Verification items for the finished model (mm, model axes). Face numbers are marked on the shaded views. A direction names the side the tool comes from. Give positions to 0.01 mm unless a question says otherwise; leave off trailing zeros. Write each loop counter-clockwise with the first axis right and the second up, starting at its lowest first coordinate (ties: lowest second). Pieces come first, ordered by that corner, then holes. Notation, with made-up numbers: M -31,18 L 25,18 A22 ccw 25,55 Z; hole C 83.5,72.25 d4. An arc over 180 degrees is marked long. Write item = value, one per line.
from build123d import *

# Parameters (mm, degrees)
STOCK_DEPTH        = 9.525
MOUNTING_HOLE_D    = 6.35
SPRING_HOLE_D      = 4.7625
FILLET3_R          = 9.525
FILLET4_R          = 1.27
SKETCH15_W         = 12.7
SKETCH15_H         = 12.7
CUT_EXTRUDE1_DEPTH = 3.175
SKETCH16_W         = 12.7
SKETCH16_H         = 12.7
CUT_EXTRUDE2_DEPTH = 3.175
FILLET5_R          = 3.175


# Some blends are built 0.0001 mm under size
with BuildPart() as part:
    # Sketch7 → Stock (new body)
    with BuildSketch(Plane(origin=(0, 0, 0), x_dir=(1, 0, 0), z_dir=(0, 1, 0))):
        Polygon((0, 0), (0, 19.05), (-7.874, 19.05), (-7.874, 28.575), (6.096, 28.575), (6.096, 69.85), (18.796, 69.85), (18.796, 28.575), (23.876, 28.575), (23.876, 0), align=None)
    extrude(amount=STOCK_DEPTH)

    # Mounting Hole (through all)
    with Locations(Plane(origin=(0, 9.525, 0), x_dir=(1, 0, 0), z_dir=(0, 1, 0))):
        with Locations((14.224, 9.525)):
            Hole(MOUNTING_HOLE_D / 2)

    # Spring Hole (through all)
    with Locations(Plane(origin=(0, 9.525, 0), x_dir=(1, 0, 0), z_dir=(0, 1, 0))):
        with Locations((12.446, 63.5)):
            Hole(SPRING_HOLE_D / 2)

    # Fillet3
    # the kernel refuses this fillet: 9.525 mm, written as the material it adds along each edge
    with BuildSketch(Plane(origin=(6.096, 0, -28.575), x_dir=(-1, 0, 0), z_dir=(0, 1, 0))) as fillet3_piece_1:
        with BuildLine():
            CenterArc((FILLET3_R, -FILLET3_R), FILLET3_R, 90, 90)
            Line((0, -FILLET3_R), (-FILLET3_R * 0.02, -FILLET3_R))
            Line((-FILLET3_R * 0.02, -FILLET3_R), (-FILLET3_R * 0.02, FILLET3_R * 0.02))
            Line((-FILLET3_R * 0.02, FILLET3_R * 0.02), (FILLET3_R, FILLET3_R * 0.02))
            Line((FILLET3_R, FILLET3_R * 0.02), (FILLET3_R, 0))
        make_face()
    extrude(amount=9.525)
    with BuildSketch(Plane(origin=(18.796, 0, -28.575), x_dir=(1, 0, 0), z_dir=(0, 1, 0))) as fillet3_piece_2:
        with BuildLine():
            CenterArc((9.525, 8.424226968), FILLET3_R, 180, 62.181860715)
            Line((0, 8.424226968), (-0.1905, 8.424226968))
            Line((-0.1905, 8.424226968), (-0.1905, 0))
            Line((-0.1905, 0), (0, -0.1905))
            ThreePointArc((0, -0.1905), (2.54, -0.1905), (4.9911, -0.168484539))
            Line((4.9911, -0.168484539), (5.08, 0))
        make_face()
    extrude(amount=9.525)

    # Fillet4
    fillet4_edges = [part.edges().sort_by_distance(p)[0] for p in [
        (-7.874, 4.7625, -28.575),
        (6.096, 4.7625, -69.85),
        (18.796, 4.7625, -69.85),
    ]]
    fillet(fillet4_edges, radius=FILLET4_R)

    # Sketch15 → Cut-Extrude1 (cut)
    with BuildSketch(Plane(origin=(0, 9.525, 0), x_dir=(1, 0, 0), z_dir=(0, 1, 0))):
        with Locations((12.446, 63.5)):
            Rectangle(SKETCH15_W, SKETCH15_H)
    extrude(amount=-CUT_EXTRUDE1_DEPTH, mode=Mode.SUBTRACT)

    # Sketch16 → Cut-Extrude2 (cut)
    with BuildSketch(Plane.XZ):
        with Locations((12.446, -63.5)):
            Rectangle(SKETCH16_W, SKETCH16_H)
    extrude(amount=-CUT_EXTRUDE2_DEPTH, mode=Mode.SUBTRACT)

    # Fillet5
    fillet5_edges = [part.edges().sort_by_distance(p)[0] for p in [
        (12.446, 3.175, -57.15),
        (12.446, 6.35, -57.15),
    ]]
    fillet(fillet5_edges, radius=FILLET5_R - 0.0001)  # a hair under: the kernel refuses the full size


solid = part.part
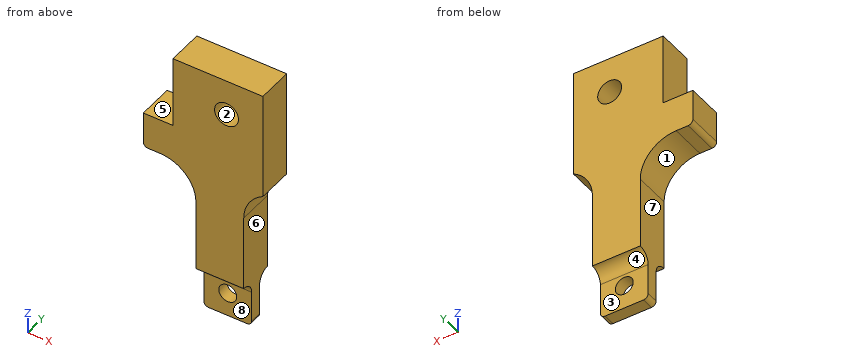
1) Material ranges on probe 1 along X at (y, z) = (5.4, -63.5); probe 2 along Z at (x, y) = (12.5, 5.5); probe 3 along X at (y, z) = (6, -48), recorded low to high. Write a range as from..to.
From the geometry:
probe_1 = 6.1..10.06, 14.83..18.8
probe_2 = -69.85..-65.88, -61.12..-12.19, -6.86..0
probe_3 = 6.1..18.8
2) Tool access check on the marked faces 4, 5, 6, 7 and 8. Record the directions out of +Z, -Z, +X, -X, +Y, -Y that give a thin tool (end or side, any length) a straight path to the whole face; none if there is none.
From the geometry:
face_4 = -Z, +X, -X, +Y
face_5 = +Z, -X, +Y, -Y
face_6 = -Z, +X, +Y, -Y
face_7 = -Z, -X, +Y, -Y
face_8 = -Z, +X, -X, -Y
3) Cross-section at D-D on z = -45.5. Record the boundary of the cut face in (x, y) (3 decimals), plus the area to 3 significant figures.
From the geometry:
outline = M 6.096,0 L 18.796,0 L 18.796,9.525 L 6.096,9.525 Z
area = 121 mm^2
4) Cross-section at C-C on y = 5. Count the separate pieces of the cut face and the enclosed holes in it, plus the area to 3 significant figures.
From the geometry:
separate_pieces = 1
enclosed_holes = 2
area = 1,260 mm^2
5) Depth check by flat-ended pin: P1, Ø5, axis at y = 3, z = -5, coming from the -X side; P2, Ø4, axis at y = 7, z = -39.5, coming from the -X side; P3, Ø3, axis at x = 13, z = -67.5, coming from the +Y side. Enter the tip coordinate at first touch or a pass-through.
From the geometry:
P1 = 0
P2 = 6.08
P3 = 6.35
6) Cross-section at A-A on z = -63.5. Record the boundary of the cut face in (x, y) (3 decimals), plus the area to 3 significant figures.
From the geometry:
outline = M 6.096,3.175 L 10.065,3.175 L 10.065,6.35 L 6.096,6.35 Z; M 14.827,3.175 L 18.796,3.175 L 18.796,6.35 L 14.827,6.35 Z
area = 25.2 mm^2
7) Draft check along Z on the marked faces 1, 2 and 3. Enter one of: +Z half, -Z half, draft (parallel to the pull), parting line (faces both ways), or undercut.
From the geometry:
face_1 = -Z half
face_2 = undercut
face_3 = draft
